For this review, take the finished solid that the model builds, in its own axes (mm). A direction names the side the tool comes from. Give positions to 0.01 mm unless a question says otherwise; leave off trailing zeros. Order: outer loops, then holes, each group sorted by start corner. A loop starts at its lowest first (then second) coordinate and runs counter-clockwise, first axis right, second up. Notation, with made-up numbers: (27.5, 58) -> (80.5, 58) arc R24 ccw to (80.5, 83) -> close; hole circle Ø10 at (8.25, 1.25). An arc over 180 degrees is marked (long way). Return JSON: item names as keys, results as strings. Group by question number.
1) Insertion check: P1, Ø10, axis at x = 41.275, y = 9.525, coming from the +Z side; P2, Ø3, axis at x = 22.5, z = 43.5, coming from the -Y side; P3, Ø10, axis at y = 26.5, z = 30.5, coming from the -X side. Each pin has a flat end and moves straight along its axis. Give the tip position at first contact, or say it passes through.
2) The part is to be moulded in two halves that separate along Y. For faces 1 (the face through (10.79, 25.31, 8.16)), 2 (the face through (25, 0, 3)), 3 (the face through (11.232, 12.202, 3.219)), say which applies: released by +Y, released by -Y, zero draft, split by the parting line, or undercut.
3) Add section C-C (x = 24). Give the boundary of the cut face in (y, z).
4) To check wall thickness, follow line 1 along Z through (x, y) = (25.4, 22.5); line 2 along X through (y, z) = (24, 63); line 3 along Z through (x, y) = (21.5, 10.5). State the ranges of each line that lie inside material, in increasing order.
5) Add section B-B (y = 10.5). Give the boundary of the cut face in (x, z), then the cut area to 3 significant figures.
6) Add section A-A (y = 16.5). Give the boundary of the cut face in (x, z), then the cut area to 3 significant figures.
7) Add section D-D (z = 56). Give the boundary of the cut face in (x, y).
8) For faces 4 (the face through (22.4, 0, 69.3)), 5 (the face through (12.7, 25, 38)), 6 (the face through (38.1, 25, 38)), list the 3-axis set-ups (+Z, -Z, +X, -X, +Y, -Y) from which the entire face can be reached by the end or side of a thin tool; tool diameter is ignored.
from build123d import *

# Parameters (mm, degrees)
F0_W      = 50.8
F0_H      = 31.75
F1_DEPTH  = 6.35
F2_R      = 3.175
F3_DEPTH  = 6.35
F4_W      = 25.4
F4_H      = 69.85
F5_DEPTH  = 12.7
F7_DEPTH  = 25.4
F8_R      = 12.7
F9_DEPTH  = 19.05
F10_R     = 6.35
F11_DEPTH = 31.75
F12_R     = 5.08
F13_W     = 12.7
F13_H     = 12.7
F14_DEPTH = 12.7
F16_DEPTH = 25.4
F17_W     = 12.7
F17_H     = 12.7
F18_DEPTH = 12.7
F20_DEPTH = 25.4


with BuildPart() as f1:
    # F0 (on Top) → F1 (new body)
    with BuildSketch(Plane.XY):
        with Locations((25.4, 15.875)):
            Rectangle(F0_W, F0_H)
    extrude(amount=F1_DEPTH)

    # F2 (on face) → F3 (cut)
    with BuildSketch(Plane.XY.offset(6.35)):
        with Locations((41.275, 9.525)):
            Circle(F2_R)
        with Locations((9.525, 9.525)):
            Circle(F2_R)
    extrude(amount=-F3_DEPTH, mode=Mode.SUBTRACT)

    # F4 (on face) → F5 (join)
    with BuildSketch(Plane(origin=(0, 31.75, 0), x_dir=(-1, 0, 0), z_dir=(0, 1, 0))):
        with Locations((-25.4, 41.275)):
            Rectangle(F4_W, F4_H)
    extrude(amount=-F5_DEPTH)

    # F6 (on face) → F7 (cut)
    with BuildSketch(Plane.XZ.offset(-19.05)):
        with BuildLine():
            ThreePointArc((25.4, 76.2), (34.3802561211, 72.4802561211), (38.1, 63.5))
            Line((38.1, 63.5), (38.1, 76.2))
            Line((38.1, 76.2), (25.4, 76.2))
        make_face()
        with BuildLine():
            ThreePointArc((12.7, 63.5), (16.4197438789, 72.4802561211), (25.4, 76.2))
            Line((25.4, 76.2), (12.7, 76.2))
            Line((12.7, 76.2), (12.7, 63.5))
        make_face()
    extrude(amount=-F7_DEPTH, mode=Mode.SUBTRACT)

    # F8 (on face) → F9 (join)
    with BuildSketch(Plane.XZ.offset(-19.05)):
        with Locations((25.4, 63.5)):
            Circle(F8_R)
    extrude(amount=F9_DEPTH)

    # F10 (on face) → F11 (cut)
    with BuildSketch(Plane.XZ):
        with Locations((25.4, 63.5)):
            Circle(F10_R)
    extrude(amount=-F11_DEPTH, mode=Mode.SUBTRACT)

    # F12
    f12_edges = [f1.edges().sort_by_distance(p)[0] for p in [
        (0, 0, 3.175),
        (50.8, 0, 3.175),
    ]]
    fillet(f12_edges, radius=F12_R)

    # F13 (on face) → F14 (join)
    with BuildSketch(Plane.YZ.offset(38.1)):
        with Locations((25.4, 12.7)):
            Rectangle(F13_W, F13_H)
    extrude(amount=F14_DEPTH)

    # F15 (on face) → F16 (cut)
    with BuildSketch(Plane.XZ.offset(-19.05)):
        with BuildLine():
            ThreePointArc((38.1, 12.7), (44.45, 6.35), (50.8, 12.7))
            ThreePointArc((50.8, 12.7), (44.45, 19.05), (38.1, 12.7))
        make_face()
        with BuildLine():
            Line((50.8, 19.05), (44.45, 19.05))
            ThreePointArc((44.45, 19.05), (48.9401280605, 17.1901280605), (50.8, 12.7))
            Line((50.8, 12.7), (50.8, 19.05))
        make_face()
        with BuildLine():
            Line((44.45, 19.05), (38.1, 19.05))
            Line((38.1, 19.05), (38.1, 12.7))
            ThreePointArc((38.1, 12.7), (39.9598719395, 17.1901280605), (44.45, 19.05))
        make_face()
        with BuildLine():
            ThreePointArc((50.8, 12.7), (48.9401280605, 8.2098719395), (44.45, 6.35))
            Line((44.45, 6.35), (50.8, 6.35))
            Line((50.8, 6.35), (50.8, 12.7))
        make_face()
    extrude(amount=-F16_DEPTH, mode=Mode.SUBTRACT)

    # F17 (on face) → F18 (join)
    with BuildSketch(Plane(origin=(12.7, 0, 0), x_dir=(0, -1, 0), z_dir=(-1, 0, 0))):
        with Locations((-25.4, 12.7)):
            Rectangle(F17_W, F17_H)
    extrude(amount=F18_DEPTH)

    # F19 (on face) → F20 (cut)
    with BuildSketch(Plane.XZ.offset(-19.05)):
        with BuildLine():
            ThreePointArc((6.35, 6.35), (10.8401280605, 8.2098719395), (12.7, 12.7))
            ThreePointArc((12.7, 12.7), (10.8401280605, 17.1901280605), (6.35, 19.05))
            ThreePointArc((6.35, 19.05), (1.8598719395, 17.1901280605), (0, 12.7))
            ThreePointArc((0, 12.7), (1.8598719395, 8.2098719395), (6.35, 6.35))
        make_face()
        with BuildLine():
            ThreePointArc((0, 12.7), (1.8598719395, 17.1901280605), (6.35, 19.05))
            Line((6.35, 19.05), (0, 19.05))
            Line((0, 19.05), (0, 12.7))
        make_face()
        with BuildLine():
            Line((0, 6.35), (6.35, 6.35))
            ThreePointArc((6.35, 6.35), (1.8598719395, 8.2098719395), (0, 12.7))
            Line((0, 12.7), (0, 6.35))
        make_face()
        with BuildLine():
            Line((12.7, 12.7), (12.7, 19.05))
            Line((12.7, 19.05), (6.35, 19.05))
            ThreePointArc((6.35, 19.05), (10.8401280605, 17.1901280605), (12.7, 12.7))
        make_face()
    extrude(amount=-F20_DEPTH, mode=Mode.SUBTRACT)


solid = f1.part
Evaluation:
{
 "1": {"P1": "z = 70.06", "P2": "y = 19.05", "P3": "x = 12.7"},
 "2": {"face 1": "zero draft", "face 2": "released by -Y", "face 3": "undercut"},
 "3": {"outline": "(0, 0) -> (31.75, 0) -> (31.75, 57.31) -> (0, 57.31) -> (0, 50.88) -> (19.05, 50.88) -> (19.05, 6.35) -> (0, 6.35) -> close; (0, 69.69) -> (31.75, 69.69) -> (31.75, 76.12) -> (0, 76.12) -> close"},
 "4": {"line 1": "0 to 57.15, 69.85 to 76.2", "line 2": "12.7 to 19.07, 31.73 to 38.1", "line 3": "0 to 6.35, 51.41 to 58.49, 68.51 to 75.59"},
 "5": {"outline": "(0, 0) -> (6.5, 0) -> (6.5, 6.35) -> (0, 6.35) -> close; (12.55, 0) -> (38.25, 0) -> (38.25, 6.35) -> (12.55, 6.35) -> close; circle Ø25.4 at (25.4, 63.5); (44.3, 0) -> (50.8, 0) -> (50.8, 6.35) -> (44.3, 6.35) -> close; hole circle Ø12.7 at (25.4, 63.5)", "area": "626 mm^2"},
 "6": {"outline": "(0, 0) -> (50.8, 0) -> (50.8, 6.35) -> (0, 6.35) -> close; circle Ø25.4 at (25.4, 63.5); hole circle Ø12.7 at (25.4, 63.5)", "area": "703 mm^2"},
 "7": {"outline": "(12.7, 19.05) -> (15.15, 19.05) -> (15.15, 0) -> (35.65, 0) -> (35.65, 19.05) -> (38.1, 19.05) -> (38.1, 31.75) -> (12.7, 31.75) -> close"},
 "8": {"face 4": "+Z, -Z, +X, -X, -Y", "face 5": "+Z, -X, +Y, -Y", "face 6": "+Z, +X, +Y, -Y"}
}
